Source: CAD feature listing. Evaluate the final solid. Frame: model axes, mm. A direction names the side the tool comes from. Round coordinates to 2 decimals unless told otherwise and drop trailing zeros. Loops run counter-clockwise (first coordinate to the right, second up) from the corner with the lowest first, then second, coordinate; pieces in that order, holes last. Notation, with made-up numbers: (74.25, 62) - (123.25, 62) arc R24 cw to (123.25, 83) - close; hole circle Ø1 at (12, 62). An arc over 180 degrees is marked (long way). One line per question, with ' | ' between items.
from build123d import *

# Parameters (mm, degrees)
F0_W     = 3
F0_H     = 3
F1_DEPTH = 3.3
F3_DEPTH = 9.7
F4_DEPTH = 25
F5_W     = 15.5733765569
F5_H     = 2.1997606382
F6_DEPTH = 9.7
F8_R     = 2


with BuildPart() as f1:
    # F0 (on Front) → F1 (new body)
    with BuildSketch(Plane.XZ):
        with BuildLine():
            Line((0, 34), (0, 0))
            Line((0, 0), (30.2820131183, 0))
            Line((30.2820131183, 0), (30.2820131183, 16.368644312))
            Line((30.2820131183, 16.368644312), (17.0356687158, 16.368644312))
            Line((17.0356687158, 16.368644312), (17.0356687158, 12.4485930428))
            Line((17.0356687158, 12.4485930428), (18.0357955396, 12.4485930428))
            Line((18.0357955396, 12.4485930428), (18.0357955396, 10.2488324046))
            Line((18.0357955396, 10.2488324046), (2.4624189828, 10.2488324046))
            Line((2.4624189828, 10.2488324046), (2.4624189828, 12.4485930428))
            Line((2.4624189828, 12.4485930428), (3.5426469985, 12.4485930428))
            Line((3.5426469985, 12.4485930428), (3.5426469985, 24.6681645513))
            add(Edge.make_bspline(
                [(6.5175484558, 29.5915287649), (6.2907197581, 29.9241725963), (5.8790854313, 30.5278335133), (5.1978575268, 30.8967943754), (3.7389888493, 30.7860278706), (3.4619052088, 28.4189645391), (3.5129095402, 26.0495961355), (3.5426469985, 24.6681645513)],
                knots=[0, 0, 0, 0, 0.1657910439, 0.3008670659, 0.4665066802, 0.6889531738, 1, 1, 1, 1], degree=3))
            Line((6.5175484558, 29.5915287649), (10.5911474675, 20.7152888179))
            Line((10.5911474675, 20.7152888179), (6.1143967323, 20.7152888179))
            Line((6.1143967323, 20.7152888179), (6.1143967323, 17.1928294003))
            Line((6.1143967323, 17.1928294003), (15.821730718, 17.1928294003))
            Line((15.821730718, 17.1928294003), (8.1083662808, 34))
            Line((8.1083662808, 34), (0, 34))
        make_face()
        with Locations((23.9732756615, 10.9485930428)):
            Rectangle(F0_W, F0_H, mode=Mode.SUBTRACT)
    extrude(amount=F1_DEPTH)

    # F2 (on face) → F3 (join)
    with BuildSketch(Plane(origin=(0, 0, 0), x_dir=(-1, 0, 0), z_dir=(0, 1, 0))):
        Polygon((-8.1085339189, 7.924452424), (-9.3574654311, 4.8816055059), (-6.0858423822, 4.7413739376), align=None)
        Polygon((-6.6248354992, 5.045762931), (-8.7793627754, 5.0320993178), (-9.0411501005, 5.0320993178), (-8.1026144326, 7.3713208549), align=None, mode=Mode.SUBTRACT)
        Polygon((-25.4732756615, 12.4485930428), (-25.4732756615, 9.4485930428), (-22.4732756615, 12.4485930428), align=None)
        Polygon((-22.9099839926, 12.2652184218), (-25.3357663751, 9.8863113672), (-25.3357663751, 12.2652184218), align=None, mode=Mode.SUBTRACT)
        Polygon((-22.4732756615, 12.4485930428), (-25.4732756615, 9.4485930428), (-22.4732756615, 9.4485930428), align=None)
        Polygon((-22.6521715522, 9.6753742546), (-25.1131094992, 9.6284989268), (-22.6521715522, 12.0894368738), align=None, mode=Mode.SUBTRACT)
    extrude(amount=-F3_DEPTH)

    # F2 (on face) → F4 (cut)
    with BuildSketch(Plane(origin=(0, 0, 0), x_dir=(-1, 0, 0), z_dir=(0, 1, 0))):
        Polygon((-9.0411501005, 5.0320993178), (-8.7793627754, 5.0320993178), (-6.6248354992, 5.045762931), (-8.1026144326, 7.3713208549), align=None)
    extrude(amount=-F4_DEPTH, mode=Mode.SUBTRACT)

    # F5 (on face) → F6 (join)
    with BuildSketch(Plane(origin=(0, 0, 0), x_dir=(-1, 0, 0), z_dir=(0, 1, 0))):
        with Locations((-10.2491072612, 11.3487127237)):
            Rectangle(F5_W, F5_H)
    extrude(amount=-F6_DEPTH)

    # F7: F1 across face


with BuildPart() as f1_1:
    add(f1.part)
    add(f1.part.mirror(Plane(origin=(10.2491072612, -9.7, 11.3487127237), x_dir=(-1, 0, 0), z_dir=(0, -1, 0))))

    # F8
    f8_edges = [f1_1.edges().sort_by_distance(p)[0] for p in [
        (30.282013, -17.75, 16.368644),
        (30.282013, -1.65, 16.368644),
        (8.108366, -17.75, 34),
        (8.108366, -1.65, 34),
        (15.821731, -17.75, 17.192829),
        (17.035669, -17.75, 16.368644),
        (17.035669, -1.65, 16.368644),
    ]]
    fillet(f8_edges, radius=F8_R)


solid = f1_1.part
1. Section query B-B, the plane x = 20. Return loops of the section in (y, z).
Worked out:
outline: (-19.4, 0) - (-16.1, 0) - (-16.1, 16.37) - (-19.4, 16.37) - close; (-3.3, 0) - (0, 0) - (0, 16.37) - (-3.3, 16.37) - close
2. Section query D-D, the plane x = 10. Return loops of the section in (y, z).
Worked out:
outline: (-19.4, 0) - (-16.1, 0) - (-16.1, 10.25) - (-3.3, 10.25) - (-3.3, 0) - (0, 0) - (0, 12.45) - (-19.4, 12.45) - close; (-19.4, 17.19) - (-16.1, 17.19) - (-16.1, 20.72) - (-19.4, 20.72) - close; (-19.4, 22) - (-16.1, 22) - (-16.1, 29.88) - (-19.4, 29.88) - close; (-3.3, 17.19) - (0, 17.19) - (0, 20.72) - (-3.3, 20.72) - close; (-3.3, 22) - (0, 22) - (0, 29.88) - (-3.3, 29.88) - close
3. Access query for faces 1 (the flat face through (12, -3.3, 10)), 2 (the flat face through (17.036, -18, 13)), 3 (the flat face through (6.114, -18, 19)), 4 (the flat face through (24, -18, 16.369)). Directions: +Z, -Z, +X, -X, +Y, -Y. A direction counts if a zero-diameter tool reaches every point of the face in a straight line with its end or side. Return the directions, or none.
Worked out:
face 1: none | face 2: +Z, +Y, -Y | face 3: +Y, -Y | face 4: +Z, +X, +Y, -Y
4. Section query C-C, the plane z = 19. Return loops of the section in (x, y).
Worked out:
outline: (0, -19.4) - (3.54, -19.4) - (3.54, -16.1) - (0, -16.1) - close; (0, -3.3) - (3.54, -3.3) - (3.54, 0) - (0, 0) - close; (6.11, -19.4) - (14.69, -19.4) - (14.69, -16.1) - (6.11, -16.1) - close; (6.11, -3.3) - (14.99, -3.3) - (14.99, 0) - (6.11, 0) - close
5. Section query A-A, the plane y = -7.5. Return loops of the section in (x, z), plus the area to 3 significant figures.
Worked out:
outline: (2.46, 10.25) - (18.04, 10.25) - (18.04, 12.45) - (2.46, 12.45) - close; (6.09, 4.74) - (9.36, 4.88) - (8.11, 7.92) - close; (22.47, 9.45) - (25.47, 9.45) - (25.47, 12.45) - (22.47, 12.45) - close; hole (6.62, 5.05) - (8.78, 5.03) - (9.04, 5.03) - (8.1, 7.37) - close; hole (22.65, 9.68) - (25.11, 9.63) - (22.65, 12.09) - close; hole (22.91, 12.27) - (25.34, 9.89) - (25.34, 12.27) - close | area: 39.6 mm2
6. Material intervals for probe 1 along Y at (x, z) = (12.5, 24); probe 2 along X at (y, z) = (-17, 11); probe 3 along Z at (x, y) = (10, -17.5), sorted ascending.
Worked out:
probe 1: y = -19.4 to -16.1, -3.3 to 0 | probe 2: x = 0 to 22.65, 23.74 to 24.2, 25.34 to 30.28 | probe 3: z = 0 to 12.45, 17.19 to 20.72, 22 to 29.88
7. Contact query for flat-ended pins moving along their axis: P1, Ø2.5, axis at y = -11.5, z = 10.5, coming from the +X side; P2, Ø1.6, axis at x = 9.5, y = -2, coming from the +Z side; P3, Ø1.6, axis at y = -2, z = 20.5, coming from the +X side. Output: stop coordinate, or through.
Worked out:
P1: stops at x = 25.47 | P2: stops at z = 32.71 | P3: stops at x = 14.67
8. Mould query, pull axis Y, two halves, no side actions, for faces 5 (the flat face through (24, -2, 16.369)), 6 (the flat face through (7.083, -9.79, 6.311)), 7 (the flat face through (12, 0, 10)). Classes: released by +Y, released by -Y, zero draft, split by the parting line, or undercut.
Worked out:
face 5: zero draft | face 6: undercut | face 7: released by +Y
